The model under review builds one solid part; all positions refer to its coordinate system, in mm. Coordinates: 2 decimals unless noted, no trailing zeros. Loops run counter-clockwise (first coordinate to the right, second up) from the corner with the lowest first, then second, coordinate; pieces in that order, holes last. Notation, with made-up numbers: (62.5, -9) - (91.5, -9) arc R11 cw to (91.5, 3) - close; hole circle Ø9 at (1, 1.5). An arc over 180 degrees is marked (long way). Answer in a Markdown table with one row per item. Add a question column.
(1) Mouldability with a two-part tool opening along Z and no side actions: class faces 1 (the flat face through (35.5, 5, -4)), 2 (the cylindrical face through (17.64, 1.32, 29.97)), 3 (the cylindrical face through (17.998, 6.306, 8.195)) as +Z half, -Z half, draft (parallel to the pull), parting line (faces both ways), or undercut.
(2) For line 1 along Y through (x, z) = (12, 0) (3 decimals); line 2 along Z through (x, y) = (16, 5); line 3 along Z through (x, y) = (10, 5.5), list the stretches that pass through material, from the lowest coordinate up.
(3) We need section B-B on z = 0. Write out the cut boundary in (x, y) (3 decimals).
(4) We need section A-A on y = 0. Write out the cut boundary in (x, z) (3 decimals).
(5) We need section C-C on x = 13. Write out the cut boundary in (y, z) (3 decimals), plus the area to 3 significant figures.
(6) For P1, Ø6, axis at y = 5.75, z = 9.96, coming from the +X side; P2, Ø8, axis at x = 13, y = 6.5, coming from the +Z side; P3, Ø1.5, axis at x = 4, z = 23.5, coming from the +Y side; P4, Ø3, axis at y = -18, z = -19, coming from the +X side, all flat-tipped, find the tip position at first contact; note any pin that passes through.
(7) We need section D-D on x = 30. Write out the cut boundary in (y, z) (3 decimals), plus the area to 3 significant figures.
from build123d import *

# Parameters (mm, degrees)
SKETCH1_R           = 30
BOSS_EXTRUDE1_DEPTH = 35.5
SKETCH2_R           = 6.125
SKETCH2_R_2         = 1.85
CUT_EXTRUDE1_DEPTH  = 56.31952639
FILLET1_R           = 10


with BuildPart() as part:
    # Sketch1 → Boss-Extrude1 (new body)
    with BuildSketch(Plane(origin=(0, 0, 0), x_dir=(0, 0, -1), z_dir=(1, 0, 0))):
        Circle(SKETCH1_R)
    extrude(amount=BOSS_EXTRUDE1_DEPTH)

    # Sketch2 → Cut-Extrude1 (cut, through all)
    with BuildSketch(Plane(origin=(35.5, 0, 0), x_dir=(0, 0, -1), z_dir=(1, 0, 0))):
        Circle(SKETCH2_R)
        with Locations((-9.959292144, 5.75)):
            Circle(SKETCH2_R_2)
        with Locations((9.959292144, 5.75)):
            Circle(SKETCH2_R_2)
        with Locations((0, -11.5)):
            Circle(SKETCH2_R_2)
    extrude(amount=-CUT_EXTRUDE1_DEPTH, mode=Mode.SUBTRACT)

    # Fillet1
    fillet1_edges = [part.edges().sort_by_distance(p)[0] for p in [
        (0, 0, 30),
        (35.5, 0, 30),
    ]]
    fillet(fillet1_edges, radius=FILLET1_R)


solid = part.part
Outcome:
| question | item | result |
|---|---|---|
| 1 | face 1 | draft |
| 1 | face 2 | parting line |
| 1 | face 3 | undercut |
| 2 | line 1 | -30 to -13.35, -9.65 to -6.125, 6.125 to 30 |
| 2 | line 2 | -29.58 to -11.65, -8.27 to -3.54, 3.54 to 8.27, 11.65 to 29.58 |
| 2 | line 3 | -29.49 to -11.79, -8.13 to -2.7, 2.7 to 8.13, 11.79 to 29.49 |
| 3 | outline | (0, -20) arc R10 ccw to (10, -30) - (25.5, -30) arc R10 ccw to (35.5, -20) - (35.5, -13.35) - (0, -13.35) - close; (0, -9.65) - (35.5, -9.65) - (35.5, -6.125) - (0, -6.125) - close; (0, 6.125) - (35.5, 6.125) - (35.5, 20) arc R10 ccw to (25.5, 30) - (10, 30) arc R10 ccw to (0, 20) - close |
| 4 | outline | (0, -20) arc R10 ccw to (10, -30) - (25.5, -30) arc R10 ccw to (35.5, -20) - (35.5, -6.125) - (0, -6.125) - close; (0, 6.125) - (35.5, 6.125) - (35.5, 20) arc R10 ccw to (25.5, 30) - (10, 30) arc R10 ccw to (0, 20) - close |
| 5 | outline | circle Ø60 at (0, 0); hole circle Ø3.7 at (-11.5, 0); hole circle Ø12.25 at (0, 0); hole circle Ø3.7 at (5.75, -9.959); hole circle Ø3.7 at (5.75, 9.959) |
| 5 | area | 2,680 mm² |
| 6 | P1 | x = 35.5 |
| 6 | P2 | z = 29.9 |
| 6 | P3 | y = 16.66 |
| 6 | P4 | x = 34.34 |
| 7 | outline | circle Ø57.861 at (0, 0); hole circle Ø3.7 at (-11.5, 0); hole circle Ø12.25 at (0, 0); hole circle Ø3.7 at (5.75, -9.959); hole circle Ø3.7 at (5.75, 9.959) |
| 7 | area | 2,480 mm² |
